```python
from build123d import *

# Parameters (mm, degrees)
F1_DEPTH = 50.8
F3_DEPTH = 177.8
F4_SIZE2 = 127
F4_SIZE  = 14.96059746


with BuildPart() as f1:
    # F0 (on Top) → F1 (new body)
    with BuildSketch(Plane.XY):
        Polygon((0, 17.2466), (0, 9.9280379058), (17.3265462716, 0), (30.099, 0), align=None)
        Polygon((-30.099, 0), (-17.3265462716, 0), (0, 9.9280379058), (0, 17.2466), align=None)
        Polygon((0, -9.9280379058), (-17.3265462716, 0), (-30.099, 0), (0, -17.2466), align=None)
        Polygon((30.099, 0), (17.3265462716, 0), (0, -9.9280379058), (0, -17.2466), align=None)
    extrude(amount=F1_DEPTH)

    # F2 (on face) → F3 (join)
    with BuildSketch(Plane.XY.offset(50.8)):
        Polygon((0, -17.2466), (30.099, 0), (0, 17.2466), (-30.099, 0), align=None)
        Polygon((-17.3265462716, 0), (0, 9.9280379058), (17.3265462716, 0), (0, -9.9280379058), align=None, mode=Mode.SUBTRACT)
        Polygon((17.3265462716, 0), (0, 9.9280379058), (-17.3265462716, 0), (0, -9.9280379058), align=None)
    extrude(amount=F3_DEPTH)

    # F4
    f4_edges = [f1.edges().sort_by_distance(p)[0] for p in [
        (15.0495, -8.6233, 228.6),
        (15.0495, 8.6233, 228.6),
        (-15.0495, 8.6233, 228.6),
        (-15.0495, -8.6233, 228.6),
    ]]
    f4_side = f1.faces().sort_by_distance((0, 0, 228.6))[0]
    chamfer(f4_edges, length=F4_SIZE, length2=F4_SIZE2, reference=f4_side)


solid = f1.part
```
Input: part model. Units: mm. Frame: model coordinates. A direction names the side the tool comes from. Give positions to 0.01 mm unless a question says otherwise; leave off trailing zeros. Write each loop counter-clockwise with the first axis right and the second up, starting at its lowest first coordinate (ties: lowest second). Pieces come first, ordered by that corner, then holes. Notation, with made-up numbers: (73, -33.5) - (83, -33.5) arc R5 cw to (83, -28.5) - close; hole circle Ø6 at (22, 13). An arc over 180 degrees is marked (long way). Write item = value, one per line. Start each with the question number.
1) Cut plane D-D (x = 26). Return loops of the section in (y, z).
2) Cut plane B-B (x = -7.5). Return loops of the section in (y, z).
3) Draft query along Y for faces 3 (the face through (15.26, 8.503, 50.089)), 4 (the face through (-8.542, -5.034, 25.044)), 5 (the face through (-8.785, 4.895, 25.044)), 6 (the face through (2, 9, 0)). Return one class per face: pulls with the +Y half, pulls with the -Y half, needs draft (parallel to the pull), parting line crosses it, or undercut.
4) Reachability of faces 1 (the face through (8.785, -4.895, 25.044)), 2 (the face through (9.902, 6.904, 135.989)) from +Z, -Z, +X, -X, +Y, -Y: full face, straight path, thin tool, end or side. Return the list, or none.
5) Pin query (flat end, axial travel): pin 1 (6 mm diameter, centred on x = -1, z = 77, fed in from -Y); pin 2 (1 mm diameter, centred on x = 10, z = 60.5, fed in from +Y); pin 3 (1.5 mm diameter, centred on y = 11, z = 111.5, fed in from +X). Return the tip coordinate at first contact, or that it passes through.
6) Material intervals for L1, parallel to X at y = -5, z = 23.5; L2, parallel to X at y = -6.5, z = 25; L3, parallel to Y at x = 11, z = 119, sorted ascending. Write a range as [from, to].
7) Cut plane C-C (z = 87.5). Return loops of the section in (x, y), and give its area (3 significant figures).
8) Cut plane A-A (y = 2.5). Return loops of the section in (x, z).
Answers follow:
q1.outline = (-2.35, 0) - (2.35, 0) - (2.35, 101.6) - (0, 118.9) - (-2.35, 101.6) - close
q2.outline = (-12.95, 0) - (-5.63, 0) - (-5.63, 50.8) - (5.63, 50.8) - (5.63, 0) - (12.95, 0) - (12.95, 101.6) - (0, 196.98) - (-12.95, 101.6) - close
q3.face_3 = pulls with the +Y half
q3.face_4 = undercut
q3.face_5 = undercut
q3.face_6 = needs draft
q4.face_1 = -Z
q4.face_2 = +Z, +X, +Y
q5.pin_1 = -17.25
q5.pin_2 = 11.8
q5.pin_3 = 9.88
q6.L1 = [-21.37, -8.6], [8.6, 21.37]
q6.L2 = [-18.76, -5.98], [5.98, 18.76]
q6.L3 = [-8.58, 8.58]
q7.outline = (-30.1, 0) - (0, -17.25) - (30.1, 0) - (0, 17.25) - close
q7.area = 1,040 mm^2
q8.outline = (-25.74, 0) - (-12.96, 0) - (-12.96, 50.8) - (12.96, 50.8) - (12.96, 0) - (25.74, 0) - (25.74, 101.6) - (0, 210.22) - (-25.74, 101.6) - close
